Check sheet for the modelled part. Datum: model origin and axes. Units: mm. Round coordinates to 2 decimals unless told otherwise and drop trailing zeros. Loops run counter-clockwise (first coordinate to the right, second up) from the corner with the lowest first, then second, coordinate; pieces in that order, holes last. Notation, with made-up numbers: (49, 29.5) -> (83, 29.5) arc R21 cw to (83, 36.5) -> close; hole circle Ø8 at (26.25, -11.75). An arc over 180 degrees is marked (long way). One line per question, with ' | ' between items.
Autodesk Inventor part; units mm, degrees
ref_plane "Work Plane1" through (2.75, 0, 0) normal (0, -1, 0) x (1, 0, 0)
ref_plane "YZ Plane" through (0, 0, 0) normal (1, 0, 0) x (0, 1, 0)
ref_plane "XZ Plane" through (0, 0, 0) normal (0, 1, 0) x (-1, 0, 0)
sketch "Sketch1" plane through (0, 0, 0) normal (0, 0, 1) x (1, 0, 0)
  line L0 (14, 1.5) -> (14, 0)
  line L1 (-3, 0) -> (14, 0)
  line L2 (-6.4, 0) -> (17.4, 0)
  line L3 (0, 1.8) -> (0, -0.3)
  line L4 (-3, 1.5) -> (-3, 0)
  line L5 (2, 1.5) -> (2, 0) construction
  line L6 (-6.4, 0) -> (17.4, 0)
  line L7 (-3, 1.5) -> (14, 1.5)
  dimension "d4" = 3
  dimension "d5" = 14
  dimension "d6" = 12
  dimension "d13" = 3
revolve "Body" add sketch "Sketch1" angle 360 about axis through (-3, 0, 0) along (1, 0, 0)
thread "Thread1"
thread "Thread2"
chamfer "Chamfer1" distance 0.3077 distance2 0.3067 1 edges at (14, -1.5, 0) measured on face at (14, -0.7567, -0.3972)
chamfer "Chamfer2" distance 0.501 distance2 0.3067 1 edges at (-3, -1.5, 0) measured on face at (8.1289, 1.4951, -0.1207)
ref_plane "Work Plane1" through (2.75, 0, 0) normal (0, -1, 0) x (1, 0, 0)
equation "\"d4\" = KOH"
equation "\"d5\" = NLG"
equation "\"d6\" = GEL"
equation "\"d13\" = GD"
equation "\"d1\" = KOH"
equation "\"d7\" = GEL + GAL"
equation "\"d10\" = -0.5 * SPD + 0.5 * GD"
equation "\"d12\" = -0.5 * SPD + 0.5 * GD"
equation "\"NLG\" = 14"
equation "\"GEL\" = 12"
equation "\"GAL\" = 0.61345 * PTC"
equation "\"SPD\" = NND - 1.2269 * PTC"
equation "\"d0\" = GD"
equation "\"GUL\" = 0.61345 * PTC"
equation "\"KOH\" = NND"
equation "\"GD\" = NND"
equation "\"BDM\" = NND"
equation "\"GUL1\" = 0.5"
equation "\"GAL1\" = 0.5"
equation "\"d80\" = -GUL - GEL"
equation "\"d86\" = -KOH + GUL1"
equation "\"PTC\" = 0.5"
equation "\"THREADDIA\" = 3"
equation "\"TOA\" = 30deg"
equation "\"NND\" = 3"
equation "\"GD1\" = THREADDIA - 1.2269 * PTC"
properties part number "CSN 02 1174 - A M3 x 14" material "Steel, Mild"
(1) Go/stop test with a flat-tipped pin: pin 1 (1.5 mm diameter, centred on x = 2, z = 1, fed in from +Y). Record where the tip stops, or that it passes through.
Answer:
pin 1: stops at y = 1.48
(2) Scan lines: probe 1 along Y at (x, z) = (2, -0.1); probe 2 along Y at (x, z) = (2, 1); probe 3 along Z at (x, y) = (0.25, 0.65). Record each from-to range of solid material in increasing order.
Answer:
probe 1: y = -1.5 to 1.5 | probe 2: y = -1.12 to 1.12 | probe 3: z = -1.35 to 1.35
(3) Sectioned sample at A-A, the plane x = 1.75. Record the cut outline in (y, z).
Answer:
outline: circle Ø3 at (0, 0)
